Drawing for the job (mm, zero at the part's lowest x, y, z). Coordinates: 2 decimals unless noted, no trailing zeros. Write each loop counter-clockwise with the first axis right and the second up, starting at its lowest first coordinate (ties: lowest second). Pieces come first, ordered by that corner, then holes. Notation, with made-up numbers: (70, 30) - (84, 30) arc R22 ccw to (84, 61) - close; hole circle Ø5 at (60, 6.5). An arc over 180 degrees is marked (long way). Write each question's results on one line, items separated by ' | '.
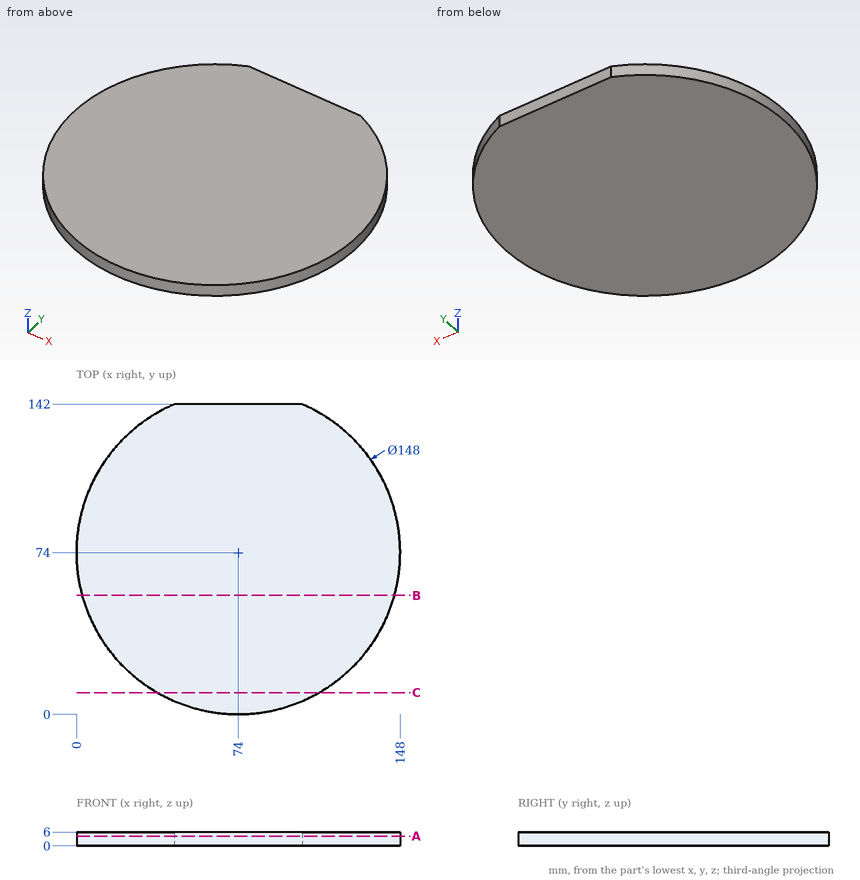
(1) Saw through at A-A on z = 4.3. Write the cut outline in (x, y).
Return value:
outline: (44.81, 142) arc R74 ccw (long way) to (103.19, 142) - close
(2) Wall check: line 1 (Y direction, x = 72, z = 2.6); line 2 (X direction, y = 72.5, z = 3.9); line 3 (Y direction, x = 41, z = 2.1). Give the ranges that are in metal, low to high. Write a range as from..to.
Return value:
line 1: y = 0.03..142 | line 2: x = 0.02..147.98 | line 3: y = 7.77..140.23
(3) Saw through at B-B on y = 54.5. Write the cut outline in (x, z), then the cut area to 3 significant figures.
Return value:
outline: (2.62, 0) - (145.38, 0) - (145.38, 6) - (2.62, 6) - close | area: 857 mm^2
(4) Saw through at C-C on y = 10. Write the cut outline in (x, z).
Return value:
outline: (36.85, 0) - (111.15, 0) - (111.15, 6) - (36.85, 6) - close
(5) Flat gauge pin, fed straight in: P1, Ø3, axis at y = 83, z = 4.5, coming from the +X side. Where does the tip first touch, or does it go through?
Return value:
P1: stops at x = 147.62
